Autodesk Inventor part; units mm, degrees
ref_plane "YZ Plane" through (0, 0, 0) normal (1, 0, 0) x (0, 1, 0)
ref_plane "XZ Plane" through (0, 0, 0) normal (0, 1, 0) x (-1, 0, 0)
ref_plane "XY Plane" through (0, 0, 0) normal (0, 0, 1) x (1, 0, 0)
sketch "Sketch1" plane through (0, 0, 0) normal (0, 1, 0) x (-1, 0, 0)
  line L0 (0, 0) -> (10, 0)
  line L1 (10, 0) -> (10, 150)
  line L2 (10, 150) -> (0, 150)
  line L3 (0, 150) -> (0, 0)
  line L4 (0, 6) -> (-34, 6)
  line L5 (-34, 6) -> (-34, 0)
  line L6 (-34, 0) -> (0, 0)
  line L7 (0, 0) -> (0, 6)
  dimension "d0" = 10
  dimension "d1" = 150
  dimension "d2" = 34
  dimension "d3" = 6
extrude "Extrusion1" add sketch "Sketch1" along normal blind 20
sketch "Sketch2" plane through (0, 0, 6) normal (0, 0, 1) x (1, 0, 0)
  circle A0 centre (25.543, 10) radius 3.1
  line L0 (34, 0) -> (34, 20)
  point P0 (0, 0)
  point P1 (34, 10)
  dimension "d6" = 6.2
  dimension "d9" = 8.457
extrude "Extrusion2" cut sketch "Sketch2" against normal through all
chamfer "Chamfer2" distance 1 angle 45 1 edges at (22.443, 10, 6)
sketch "Sketch3" plane through (0, 0, 6) normal (0, 0, 1) x (1, 0, 0)
  line L0 (34, 0) -> (34, 20)
  line L1 (34, 5) -> (13, 0)
  line L2 (34, 0) -> (-10, 0)
  line L3 (34, 15) -> (13, 20)
  line L4 (0, 20) -> (34, 20)
  line L5 (34, 0) -> (34, 20)
  circle A0 centre (25.543, 10) radius 3.1
  point P0 (0, 0)
  point P1 (34, 15)
  dimension "d16" = 10
  dimension "d17" = 5
  dimension "d18" = 21
extrude "Extrusion3" cut sketch "Sketch3" against normal through all contours L2 L1 L0 | L3 L4 L0
fillet "Fillet1" radius 4 4 edges at (34, 5, 3) (34, 15, 3) (13, 20, 3) (13, 0, 3)
chamfer "Chamfer3" distance 15 angle 45 1 edges at (0, 10, 6)
equation "\"d17\" = 0.5 * d16"
properties part number "rotator_squarer"
Build history of the part. All positions in model axes, mm. A direction names the side the tool comes from. Round coordinates to 2 decimals unless told otherwise and drop trailing zeros. Loops run counter-clockwise (first coordinate to the right, second up) from the corner with the lowest first, then second, coordinate; pieces in that order, holes last. Notation, with made-up numbers: (78.25, 38) -> (129.25, 38) arc R23 cw to (129.25, 71) -> close; hole circle Ø5 at (62.5, -35). An arc over 180 degrees is marked (long way). Use CSV: the item, a comma, the result in double quotes. Start each with the question number.
Q1. Mould opens along Y. For faces 1 (the face through (28.5, 10.93, 2.54)), 2 (the face through (33.16, 5.71, 2.96)), 3 (the face through (-4, 20, 76)), 4 (the face through (20, 10, 6)) say: +Y half, -Y half, draft (parallel to the pull), parting line (faces both ways), or undercut.
Q2. Saw through at B-B on y = 1.75. Give the cut face in (x, z).
Q3. Saw through at C-C on x = 11. Give the cut face in (y, z), and give its area (3 significant figures).
Q4. Drill centre lines: L1, parallel to Z at x = 21, y = 12; L2, parallel to X at y = 3.5, z = 84; L3, parallel to Z at x = 12, y = 10. Where is each one in solid material? Low to high.
Q5. Flat gauge pins, fed straight in: pin 1 Ø8 at (x, y) = (8, 3) entering from +Z; pin 2 Ø5.5 at (x, y) = (22.5, 7) entering from +Z; pin 3 Ø10 at (y, z) = (6.5, 63.5) entering from +X; pin 4 Ø1 at (x, y) = (25.5, 8) entering from +Z. Where does each tip first touch, or does it go through?
Q6. Saw through at D-D on z = 110. Give the cut face in (x, y).
Q7. Saw through at A-A on y = 10. Give the cut face in (x, z), and give its area (3 significant figures).
Q8. Which spindle directions (+Z, -Z, +X, -X, +Y, -Y) get a long thin tool onto all of the face, cutting with end or side? Do faces 5 (the face through (33.116, 14.349, 2.958)), 6 (the face through (0, 10, 86)). Say none if no direction does.
Solutions:
1,face 1,"undercut"
1,face 2,"-Y half"
1,face 3,"+Y half"
1,face 4,"draft"
2,outline,"(-10, 0) -> (20.35, 0) -> (20.35, 6) -> (15, 6) -> (0, 21) -> (0, 150) -> (-10, 150) -> close"
3,outline,"(0, 0) -> (20, 0) -> (20, 10) -> (0, 10) -> close"
3,area,"200 mm^2"
4,L1,"z = 0 to 6"
4,L2,"x = -10 to 0"
4,L3,"z = 0 to 9"
5,pin 1,"stops at z = 17"
5,pin 2,"stops at z = 6"
5,pin 3,"stops at x = 0"
5,pin 4,"passes through"
6,outline,"(-10, 0) -> (0, 0) -> (0, 20) -> (-10, 20) -> close"
7,outline,"(-10, 0) -> (22.44, 0) -> (22.44, 5) -> (21.44, 6) -> (15, 6) -> (0, 21) -> (0, 150) -> (-10, 150) -> close; (28.64, 0) -> (34, 0) -> (34, 6) -> (29.64, 6) -> (28.64, 5) -> close"
7,area,"1,780 mm^2"
8,face 5,"+Z, -Z, +X, +Y"
8,face 6,"+Z, +X, +Y, -Y"
